```python
from build123d import *

# Parameters (mm, degrees)
SKETCH1_R           = 10
BOSS_EXTRUDE1_DEPTH = 15
SKETCH2_R           = 9
SKETCH2_R_2         = 4
CUT_EXTRUDE1_DEPTH  = 1
SKETCH3_R           = 1.7
CUT_EXTRUDE2_DEPTH  = 4


with BuildPart() as part:
    # Sketch1 → Boss-Extrude1 (new body)
    with BuildSketch(Plane(origin=(0, 0, 0), x_dir=(1, 0, 0), z_dir=(0, 1, 0))):
        with Locations(Location((0, 0, 0), (0, 0, 270))):
            Circle(SKETCH1_R)
    extrude(amount=BOSS_EXTRUDE1_DEPTH)

    # Sketch2 → Cut-Extrude1 (cut)
    with BuildSketch(Plane(origin=(0, 15, 0), x_dir=(1, 0, 0), z_dir=(0, 1, 0))):
        with Locations(Location((0, 0, 0), (0, 0, 270))):
            Circle(SKETCH2_R)
        with Locations(Location((0, 0, 0), (0, 0, 270))):
            Circle(SKETCH2_R_2, mode=Mode.SUBTRACT)
    extrude(amount=-CUT_EXTRUDE1_DEPTH, mode=Mode.SUBTRACT)

    # Sketch3 → Cut-Extrude2 (cut)
    with BuildSketch(Plane.XZ):
        with Locations(Location((0, 0, 0), (0, 0, 270))):
            Circle(SKETCH3_R)
    extrude(amount=-CUT_EXTRUDE2_DEPTH, mode=Mode.SUBTRACT)


solid = part.part
```
For this review, take the finished solid that the model builds, in its own axes (mm). A direction names the side the tool comes from. Coordinates: 2 decimals unless noted, no trailing zeros. Write each loop counter-clockwise with the first axis right and the second up, starting at its lowest first coordinate (ties: lowest second). Pieces come first, ordered by that corner, then holes.
(1) Tool access review of faces 1 (the face through (0, 4, 0)), 2 (the face through (-2, 14, 4)), 3 (the face through (0, 15, 0)): name each direction out of +Z, -Z, +X, -X, +Y, -Y from which nothing blocks a thin tool from reaching the whole face with its end or side.
(2) The part is to be moulded in two halves that separate along X. For faces 4 (the face through (0, 0, 2)), 5 (the face through (2.703, 14.507, 8.584)), 6 (the face through (-9.76, 7.4, -2.17)), say which applies: +X half, -X half, draft (parallel to the pull), parting line (faces both ways), or undercut.
(3) Add section B-B on x = 0. Give the boundary of the cut face in (y, z).
(4) Add section A-A on z = 0. Give the boundary of the cut face in (x, y).
(5) For pin 1 Ø1 at (x, y) = (-4, 10.5) entering from -Z; pin 2 Ø5 at (y, z) = (7.5, -0.5) entering from -X; pin 3 Ø2.5 at (x, z) = (0, 0) entering from -Y; pin 4 Ø3 at (x, z) = (4, -4.5) entering from +Y, all flat-tipped, find the tip position at first contact; note any pin that passes through.
(6) Wall thickness on probe 1 along X at (y, z) = (1.35, 0); probe 2 along X at (y, z) = (14.6, 0); probe 3 along Y at (x, z) = (3.25, -2.5): over which ranges is each line inside the solid? List them lowest first.
(7) Add section C-C on y = 9. Give the boundary of the cut face in (x, z), then the cut area to 3 significant figures.
(8) Add section D-D on y = 3.5. Give the boundary of the cut face in (x, z).
Answer sheet:
1. face 1: -Y
1. face 2: +Y
1. face 3: +Z, -Z, +X, -X, +Y
2. face 4: draft
2. face 5: undercut
2. face 6: parting line
3. outline: (0, -10) - (15, -10) - (15, -9) - (14, -9) - (14, -4) - (15, -4) - (15, 4) - (14, 4) - (14, 9) - (15, 9) - (15, 10) - (0, 10) - (0, 1.7) - (4, 1.7) - (4, -1.7) - (0, -1.7) - close
4. outline: (-10, 0) - (-1.7, 0) - (-1.7, 4) - (1.7, 4) - (1.7, 0) - (10, 0) - (10, 15) - (9, 15) - (9, 14) - (4, 14) - (4, 15) - (-4, 15) - (-4, 14) - (-9, 14) - (-9, 15) - (-10, 15) - close
5. pin 1: stops at z = -9.37
5. pin 2: stops at x = -10
5. pin 3: stops at y = 4
5. pin 4: stops at y = 14
6. probe 1: x = -10 to -1.7, 1.7 to 10
6. probe 2: x = -10 to -9, -4 to 4, 9 to 10
6. probe 3: y = 0 to 14
7. outline: circle Ø20 at (0, 0)
7. area: 314 mm2
8. outline: circle Ø20 at (0, 0); hole circle Ø3.4 at (0, 0)
